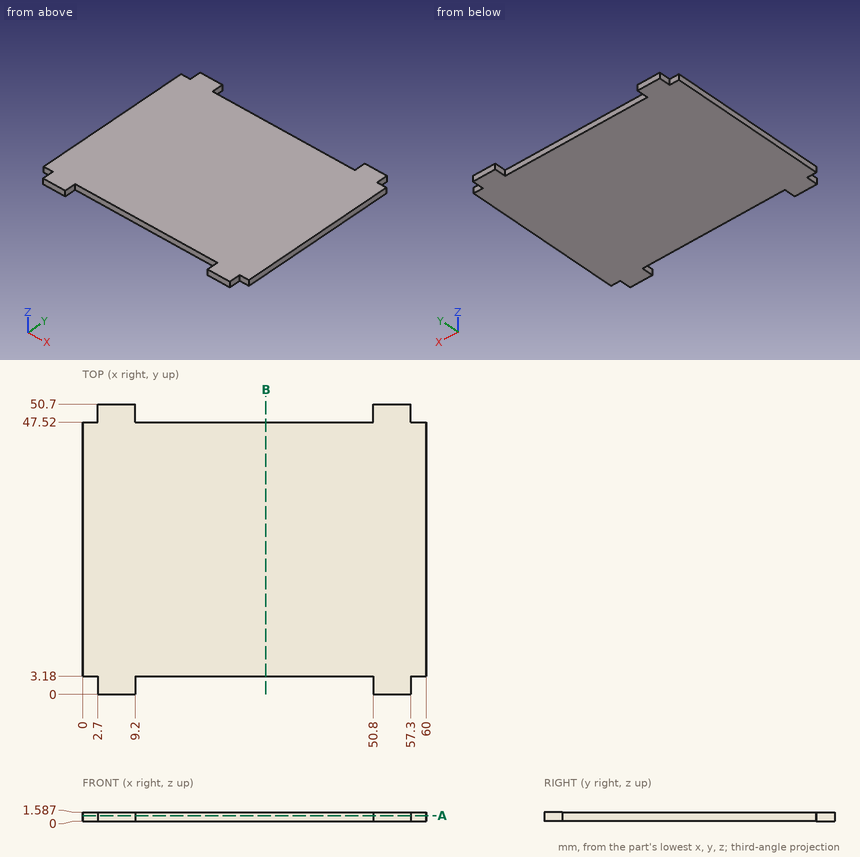
Can you work these out from the drawing? Everything is in mm from the part's minimum corner. Coordinates: 2 decimals unless noted, no trailing zeros. Loops run counter-clockwise (first coordinate to the right, second up) from the corner with the lowest first, then second, coordinate; pieces in that order, holes last.
1. For P1, Ø0.5, axis at x = 22, z = 0.5, coming from the -Y side; P2, Ø0.8, axis at y = 1.5, z = 0.5, coming from the -X side; P3, Ø0.5, axis at x = 0.5, z = 1, coming from the +Y side, each with a flat end and sliding along its axis, tell me the tip position at first contact or that it passes through.
2. Imagine slicing it at B-B, the plane x = 32. Please give me the cut outline in (y, z).
3. Imagine slicing it at A-A, the plane z = 1. Please give me the cut outline in (x, y).
4. I need wall thicknesses on L1, parallel to X at y = 48, z = 1.5; L2, parallel to Y at x = 17.5, z = 1.45. Which ranges of each line are inside material? Lowest first, please.
Taken from the geometry:
1. P1: stops at y = 3.18
1. P2: stops at x = 2.7
1. P3: stops at y = 47.52
2. outline: (3.18, 0) - (47.52, 0) - (47.52, 1.59) - (3.18, 1.59) - close
3. outline: (0, 3.18) - (2.7, 3.18) - (2.7, 0) - (9.2, 0) - (9.2, 3.18) - (50.8, 3.18) - (50.8, 0) - (57.3, 0) - (57.3, 3.18) - (60, 3.18) - (60, 47.52) - (57.3, 47.52) - (57.3, 50.7) - (50.8, 50.7) - (50.8, 47.52) - (9.2, 47.52) - (9.2, 50.7) - (2.7, 50.7) - (2.7, 47.52) - (0, 47.52) - close
4. L1: x = 2.7 to 9.2, 50.8 to 57.3
4. L2: y = 3.18 to 47.52
